```python
from build123d import *

# Parameters (mm, degrees)
F0_W     = 23
F0_H     = 28
F1_DEPTH = 1.5
F2_W     = 2.5
F2_H     = 13
F2_H_2   = 18
F3_DEPTH = 8.5
F4_W     = 2
F4_H     = 16
F4_H_2   = 11
F5_DEPTH = 8
F6_W     = 11.023622
F6_H     = 7.782471
F7_DEPTH = 1.5


with BuildPart() as f1:
    # F0 (on Top) → F1 (new body)
    with BuildSketch(Plane.XY):
        Rectangle(F0_W, F0_H)
    extrude(amount=F1_DEPTH)

    # F2 (on face) → F3 (join)
    with BuildSketch(Plane.XY.offset(1.5)):
        with Locations((-10.25, 7.5)):
            Rectangle(F2_W, F2_H)
        with Locations((10.25, 5)):
            Rectangle(F2_W, F2_H_2)
    extrude(amount=F3_DEPTH)

    # F4 (on face) → F5 (join)
    with BuildSketch(Plane(origin=(0, 0, 0), x_dir=(1, 0, 0), z_dir=(0, 0, -1))):
        with Locations((10.5, -6)):
            Rectangle(F4_W, F4_H)
        with Locations((-10.5, -8.5)):
            Rectangle(F4_W, F4_H_2)
    extrude(amount=F5_DEPTH)

    # F6 (on face) → F7 (join)
    with BuildSketch(Plane.XY.offset(1.5)):
        with Locations((0, -6.526084)):
            Rectangle(F6_W, F6_H)
    extrude(amount=F7_DEPTH)


solid = f1.part
```
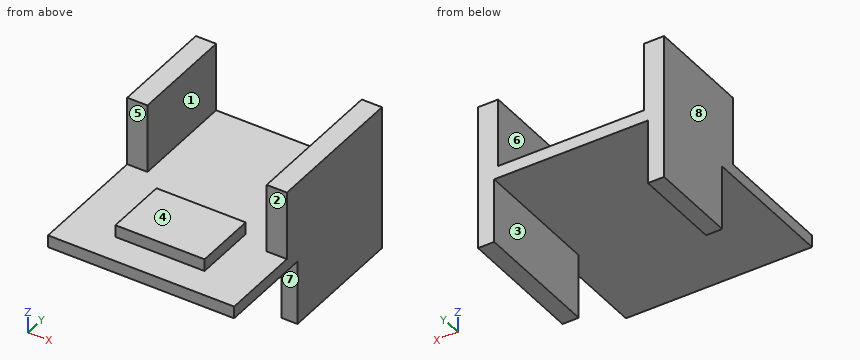
CAD build for the part. Positions are in the model's coordinates, mm. Face numbers are marked on the shaded views. A direction names the side the tool comes from. Coordinates: 2 decimals unless noted, no trailing zeros. Order: outer loops, then holes, each group sorted by start corner. A loop starts at its lowest first (then second) coordinate and runs counter-clockwise, first axis right, second up.
(1) Saw through at C-C, the plane x = 3.5. Write the cut outline in (y, z), and give its area (3 significant figures).
Solution:
outline: (-14, 0) - (14, 0) - (14, 1.5) - (-2.63, 1.5) - (-2.63, 3) - (-10.42, 3) - (-10.42, 1.5) - (-14, 1.5) - close
area: 53.7 mm2
(2) Pin check, flat tips, straight feed: pin 1 Ø0.8 at (x, z) = (10, 7.5) entering from -Y; pin 2 Ø7 at (x, y) = (4.5, 2) entering from +Z; pin 3 Ø0.8 at (x, z) = (1.5, 2) entering from -Y; pin 4 Ø6 at (y, z) = (-5, 4.5) entering from +X. Stop position of each tip, or through.
Solution:
pin 1: stops at y = -4
pin 2: stops at z = 1.5
pin 3: stops at y = -10.42
pin 4: stops at x = 11.5
(3) Drill centre lines: L1, parallel to X at y = 1.75, z = 6; L2, parallel to Z at x = 6.75, y = 11.5; L3, parallel to Y at x = 9.75, z = 6.5. Where is each one in solid material? Low to high.
Solution:
L1: x = -11.5 to -9, 9 to 11.5
L2: z = 0 to 1.5
L3: y = -4 to 14
(4) Mould opens along X. For the marked faces 6, 7 and 8 say: released by +X, released by -X, zero draft, split by the parting line, or undercut.
Solution:
face 6: undercut
face 7: zero draft
face 8: released by -X
(5) Saw through at A-A, the plane z = 4.75. Write the cut outline in (x, y), and give its area (3 significant figures).
Solution:
outline: (-11.5, 1) - (-9, 1) - (-9, 14) - (-11.5, 14) - close; (9, -4) - (11.5, -4) - (11.5, 14) - (9, 14) - close
area: 77.5 mm2
(6) Saw through at B-B, the plane z = 2.25. Write the cut outline in (x, y).
Solution:
outline: (-11.5, 1) - (-9, 1) - (-9, 14) - (-11.5, 14) - close; (-5.51, -10.42) - (5.51, -10.42) - (5.51, -2.63) - (-5.51, -2.63) - close; (9, -4) - (11.5, -4) - (11.5, 14) - (9, 14) - close
(7) Saw through at D-D, the plane y = 9.5. Write the cut outline in (x, z), and give its area (3 significant figures).
Solution:
outline: (-11.5, -8) - (-9.5, -8) - (-9.5, 0) - (9.5, 0) - (9.5, -8) - (11.5, -8) - (11.5, 10) - (9, 10) - (9, 1.5) - (-9, 1.5) - (-9, 10) - (-11.5, 10) - close
area: 109 mm2
(8) Which spindle directions (+Z, -Z, +X, -X, +Y, -Y) get a long thin tool onto all of the face, cutting with end or side? Do the marked faces 1, 2, 3, 4 and 5. Say none if no direction does.
Solution:
face 1: +Z, +Y, -Y
face 2: +Z, +X, -Y
face 3: -Z, +Y, -Y
face 4: +Z, -X, +Y, -Y
face 5: +Z, -X, -Y
